Verification items for the finished model (mm, model axes). A direction names the side the tool comes from. Round coordinates to 2 decimals unless told otherwise and drop trailing zeros. One line per item, written item: value. Start each with the question number.
Autodesk Inventor part; units mm, degrees
ref_plane "Work Plane1" through (0, 0, 0.5) normal (0, 0, -1) x (-1, 0, 0)
ref_plane "Work Plane2" through (0, 0, 0.8) normal (0, 0, -1) x (-1, 0, 0)
ref_plane "Work Plane3" through (0, 0, 1.3) normal (0, 0, -1) x (-1, 0, 0)
sketch "Sketch1" plane through (0, 0, 0) normal (0, 0, 1) x (1, 0, 0)
  line L0 (-25, 2) -> (-25, -2)
  line L1 (0, 0.3189) -> (0, -1.0844) construction
  line L2 (-25, 2) -> (25, 2)
  line L3 (25, 2) -> (25, -2)
  line L4 (25, -2) -> (-25, -2)
  line L5 (-1.8046, 0) -> (4.5195, 0) construction
  arc A0 (-23.4, 2) -> (-21.6, 2) centre (-22.5, 2) ccw
  arc A1 (-20.025, 2) -> (-15.975, 2) centre (-18, 2) ccw
  arc A2 (-15.525, 2) -> (-11.475, 2) centre (-13.5, 2) ccw
  arc A3 (-11.025, 2) -> (-6.975, 2) centre (-9, 2) ccw
  arc A4 (-5.4, 2) -> (-3.6, 2) centre (-4.5, 2) ccw
  arc A5 (-2.025, 2) -> (2.025, 2) centre (0, 2) ccw
  arc A6 (2.475, 2) -> (6.525, 2) centre (4.5, 2) ccw
  arc A7 (6.975, 2) -> (11.025, 2) centre (9, 2) ccw
  arc A8 (11.475, 2) -> (15.525, 2) centre (13.5, 2) ccw
  arc A9 (17.125, 2) -> (18.875, 2) centre (18, 2) ccw
  arc A10 (21.625, 2) -> (23.375, 2) centre (22.5, 2) ccw
  arc A11 (-18.225, -2) -> (-22.275, -2) centre (-20.25, -2) ccw
  arc A12 (-13.725, -2) -> (-17.775, -2) centre (-15.75, -2) ccw
  arc A13 (-9.225, -2) -> (-13.275, -2) centre (-11.25, -2) ccw
  arc A14 (-4.725, -2) -> (-8.775, -2) centre (-6.75, -2) ccw
  arc A15 (-2.535, -2) -> (-4.255, -2) centre (-3.395, -2) ccw
  arc A16 (-0.245, -2) -> (-1.965, -2) centre (-1.105, -2) ccw
  arc A17 (4.275, -2) -> (0.225, -2) centre (2.25, -2) ccw
  arc A18 (8.775, -2) -> (4.725, -2) centre (6.75, -2) ccw
  arc A19 (13.275, -2) -> (9.225, -2) centre (11.25, -2) ccw
  arc A20 (17.775, -2) -> (13.725, -2) centre (15.75, -2) ccw
  arc A21 (20.675, -2) -> (18.925, -2) centre (19.8, -2) ccw
  arc A22 (23.375, -2) -> (21.625, -2) centre (22.5, -2) ccw
  point P0 (0, 0)
  dimension "d0" = 4
  dimension "d1" = 50
  dimension "d2" = 2.5
  dimension "d3" = 4.5
  dimension "d4" = 4.5
  dimension "d5" = 4.5
  dimension "d6" = 4.5
  dimension "d7" = 4.5
  dimension "d8" = 4.5
  dimension "d10" = 4.5
  dimension "d11" = 4.5
  dimension "d12" = 4.5
  dimension "d13" = 4.5
  dimension "d14" = 1.8
  dimension "d15" = 4.05
  dimension "d16" = 4.05
  dimension "d17" = 4.05
  dimension "d18" = 1.8
  dimension "d19" = 4.05
  dimension "d20" = 4.05
  dimension "d21" = 4.05
  dimension "d22" = 4.05
  dimension "d23" = 1.75
  dimension "d24" = 1.75
  dimension "d25" = 4.05
  dimension "d27" = 4.5
  dimension "d28" = 4.5
  dimension "d29" = 4.5
  dimension "d30" = 3.355
  dimension "d31" = 2.29
  dimension "d32" = 3.355
  dimension "d33" = 4.5
  dimension "d34" = 4.5
  dimension "d35" = 4.5
  dimension "d37" = 1.75
  dimension "d38" = 4.05
  dimension "d39" = 4.05
  dimension "d40" = 4.05
  dimension "d41" = 4.05
  dimension "d42" = 1.72
  dimension "d43" = 1.72
  dimension "d44" = 4.05
  dimension "d45" = 4.05
  dimension "d46" = 4.05
  dimension "d47" = 1.75
  dimension "d48" = 2.7
  dimension "d136" = 2.5
  dimension "d143" = 4.05
extrude "Extrusion1" add sketch "Sketch1" along normal blind 12 contours L2 A0 A1 A2 A3 A4 A5 A6 A7 A8 A9 A10 L3 L4 A22 A21 A20 A19 A18 A17 A16 A15 A14 A13 A12 A11 L0
sketch "Sketch2" plane through (23.375, 2, 0) normal (0, 1, 0) x (1, 0, 0)
  circle A0 centre (3.025, -9.9997) radius 2
  line L0 (1.625, 0) -> (1.625, -12)
  line L1 (1.625, -12) -> (1.625, -11.428)
  point P0 (-23.375, 0)
  dimension "d51" = 4
  dimension "d52" = 0.572
  dimension "d55" = 1.4
extrude "Extrusion2" cut sketch "Sketch2" against normal blind 12.5
sketch "Sketch3" plane through (-25, 2, 0) normal (0, 1, 0) x (1, 0, 0)
  circle A0 centre (-1.4, -9.9997) radius 2
  line L0 (0, 0) -> (0, -12)
  line L1 (0, -12) -> (0, -11.428)
  point P0 (25, 0)
  dimension "d58" = 4
  dimension "d59" = 0.572
  dimension "d60" = 1.4
extrude "Extrusion3" cut sketch "Sketch3" against normal blind 12.5
sketch "Sketch4" plane through (0, 0, 12) normal (0, 0, 1) x (1, 0, 0)
  line L0 (-22.4782, 2) -> (21.8218, 2)
  line L1 (21.8218, 2) -> (21.8218, 1.825)
  line L2 (21.8218, 1.825) -> (-22.4782, 1.825)
  line L3 (-22.4782, 1.825) -> (-22.4782, 2)
  line L4 (-20.025, 2) -> (-21.6, 2)
  line L5 (-25, 2) -> (-25, -2)
  line L6 (13.275, -2) -> (13.725, -2)
  line L7 (-21.5, -2) -> (-8, -2)
  line L8 (-8, -2) -> (-8, -1.825)
  line L9 (-8, -1.825) -> (-21.5, -1.825)
  line L10 (-21.5, -1.825) -> (-21.5, -2)
  line L11 (0.89, -2) -> (21.8842, -2)
  line L12 (21.8842, -2) -> (21.8842, -1.825)
  line L13 (21.8842, -1.825) -> (0.89, -1.825)
  line L14 (0.89, -1.825) -> (0.89, -2)
  line L15 (-13.725, -2) -> (-13.275, -2)
  line L16 (25, -2) -> (25, 2)
  point P0 (0, 0)
  point P1 (-20.8125, 2)
  point P2 (13.5, -2)
  point P3 (-13.5, -2)
  dimension "d63" = 0.175
  dimension "d64" = 44.3
  dimension "d65" = 2.5218
  dimension "d69" = 0.175
  dimension "d70" = 0.175
  dimension "d71" = 3.5
  dimension "d72" = 17
  dimension "d73" = 3.1158
  dimension "d74" = 24.11
extrude "Extrusion4" cut sketch "Sketch4" against normal blind 12.5
ref_plane "Work Plane1" through (0, 0, 0.5) normal (0, 0, -1) x (-1, 0, 0)
sketch "Sketch5" plane through (0, 0, 0.5) normal (0, 0, -1) x (-1, 0, 0)
  line L0 (25, 2) -> (25, -2)
  line L1 (25, 2) -> (25, 3.5)
  line L2 (25, 3.5) -> (24.5, 3.5)
  line L3 (24.5, 3.5) -> (24.1998, 2.7996)
  line L4 (24.1998, 2.7996) -> (24.3998, 2.7996)
  line L5 (24.3998, 2.7996) -> (24.3998, 2)
  line L6 (23.4, 2) -> (25, 2)
  line L7 (25, -2) -> (22.275, -2)
  line L8 (25, -2) -> (25, -3.5)
  line L9 (25, -3.5) -> (24.5, -3.5)
  line L10 (24.5, -3.5) -> (24.1998, -2.7996)
  line L11 (24.1998, -2.7996) -> (24.3998, -2.7996)
  line L12 (24.3998, -2.7996) -> (24.3998, -2)
  line L13 (0, 0) -> (0, 7.5844) construction
  line L14 (25, 2) -> (24.3998, 2)
  line L15 (25, -2) -> (24.3998, -2)
  line L16 (-25, 2) -> (-25, -2)
  line L17 (-25, 2) -> (-25, 3.5)
  line L18 (-25, 3.5) -> (-24.5, 3.5)
  line L19 (-24.5, 3.5) -> (-24.1998, 2.7996)
  line L20 (-24.1998, 2.7996) -> (-24.3998, 2.7996)
  line L21 (-24.3998, 2.7996) -> (-24.3998, 2)
  line L22 (-23.4, 2) -> (-25, 2)
  line L23 (-25, -2) -> (-22.275, -2)
  line L24 (-25, -2) -> (-25, -3.5)
  line L25 (-25, -3.5) -> (-24.5, -3.5)
  line L26 (-24.5, -3.5) -> (-24.1998, -2.7996)
  line L27 (-24.1998, -2.7996) -> (-24.3998, -2.7996)
  line L28 (-24.3998, -2.7996) -> (-24.3998, -2)
  line L29 (-25, 2) -> (-24.3998, 2)
  line L30 (-25, -2) -> (-24.3998, -2)
  dimension "d78" = 1.5
  dimension "d79" = 0.5
  dimension "d80" = 0.762
  dimension "d81" = 0.2
  dimension "d83" = 113.2
  dimension "d84" = 0.7996
  dimension "d85" = 1.5
  dimension "d86" = 0.5
  dimension "d87" = 113.2
  dimension "d88" = 0.2
  dimension "d89" = 0.762
extrude "Extrusion5" add sketch "Sketch5" against normal blind 6 contours L8 L9 L10 L11 L12 L7 | L6 L5 L4 L3 L2 L1
ref_plane "Work Plane2" through (0, 0, 0.8) normal (0, 0, -1) x (-1, 0, 0)
sketch "Sketch8" plane through (0, 0, 0.8) normal (0, 0, -1) x (-1, 0, 0)
  line L0 (25, 2) -> (25, 3.5)
  line L1 (25, 3.5) -> (24.5, 3.5)
  line L2 (24.5, 3.5) -> (24.1998, 2.7996)
  line L3 (24.1998, 2.7996) -> (24.3998, 2.7996)
  line L4 (24.3998, 2.7996) -> (24.3998, 2)
  line L5 (24.25, 2) -> (25, 2)
  line L6 (25, 2) -> (24.3998, 2)
  arc A0 (-2.0174, 1.825) -> (2.0174, 1.825) centre (0, 2) ccw
  line L7 (0, 2) -> (0, 7.911) construction
  line L8 (-24.25, 2) -> (-25, 2)
  line L9 (-25, 2) -> (-24.3998, 2)
  line L10 (-24.1998, 2.7996) -> (-24.3998, 2.7996)
  line L11 (-24.3998, 2.7996) -> (-24.3998, 2)
  line L12 (-25, 2) -> (-25, 3.5)
  line L13 (-25, 3.5) -> (-24.5, 3.5)
  line L14 (-24.5, 3.5) -> (-24.1998, 2.7996)
  point P0 (0, 0)
  dimension "d112" = 1.5
  dimension "d113" = 0.5
  dimension "d114" = 0.762
  dimension "d115" = 0.2
  dimension "d116" = 113.2
  dimension "d117" = 0.7996
extrude "Extrusion8" add sketch "Sketch8" against normal blind 6 contours L8 L12 L13 L14 L10 L11
mirror "Mirror1" about plane through (0, 0, 0) normal (0, 1, 0) of "Extrusion8"
ref_plane "Work Plane3" through (0, 0, 1.3) normal (0, 0, -1) x (-1, 0, 0)
sketch "Sketch11" plane through (0, 0, 0) normal (0, 0, -1) x (-1, 0, 0)
  line L0 (-25, 2) -> (-24.4, 2)
  line L1 (-23.375, -2) -> (-25, -2)
  line L2 (-25, 2) -> (-24, 2)
  line L3 (-24, 2) -> (-24, -2)
  line L4 (-24, -2) -> (-25, -2)
  line L5 (-25, -2) -> (-25, 2)
  line L6 (25, 2) -> (25, -2)
  line L7 (25, -2) -> (22.275, -2)
  line L8 (25, 2) -> (24, 2)
  line L9 (24, 2) -> (24, -2)
  line L10 (24, -2) -> (25, -2)
  line L11 (25, -2) -> (25, 2)
  point P0 (0, 0)
  dimension "d145" = 1
  dimension "d146" = 1
extrude "Extrusion11" add sketch "Sketch11" along normal blind 2.005
fillet "Fillet1" radius 0.5 2 edges at (24, 0, 0) (-24, 0, 0)
sketch "Sketch12" plane through (0, 0, -2.005) normal (0, 0, -1) x (-1, 0, 0)
  line L0 (-25, 2) -> (-25, -2)
  line L1 (-24, -2) -> (-24, 2)
  line L2 (-25, 0.9) -> (-24, 0.9)
  line L3 (-24, 0.9) -> (-24, -0.8147)
  line L4 (-24, -0.8147) -> (-25, -0.8147)
  line L5 (-25, -0.8147) -> (-25, 0.9)
  line L6 (-24, 2) -> (-25, 2)
  line L7 (-23.375, -2) -> (-25, -2)
  line L8 (-25, -2) -> (-24, -2)
  line L9 (-24, -2) -> (-24, -0.9)
  line L10 (-24, -0.9) -> (-25, -0.9)
  line L11 (-25, -0.9) -> (-25, -2)
  line L12 (25, -2) -> (25, 2)
  line L13 (25, 2) -> (24, 2)
  line L14 (24, 2) -> (24, 0.9)
  line L15 (24, 0.9) -> (25, 0.9)
  line L16 (25, 0.9) -> (25, 2)
  line L17 (25, -2) -> (25, -3.5)
  line L18 (25, -2) -> (24, -2)
  line L19 (24, -2) -> (24, -0.9)
  line L20 (24, -0.9) -> (25, -0.9)
  line L21 (25, -0.9) -> (25, -2)
  point P0 (0, 0)
  dimension "d150" = 1.1
  dimension "d151" = 1.1
  dimension "d152" = 1
  dimension "d153" = 1.1
  dimension "d154" = 1
  dimension "d155" = 1.1
extrude "Extrusion12" add sketch "Sketch12" along normal blind 2 contours L6 L1 L2 L0 | L4 L1 L10 L0 | L10 L1 L7 L0 | L18 L19 L20 L12 | L15 L14 L13 L12
sketch "Sketch13" plane through (25, -2, 8.5714) normal (1, 0, 0) x (0, 0, -1)
  line L0 (12.5764, 0) -> (12.5764, 1.1853)
  line L1 (12.5764, 1.1853) -> (10.5764, 1.1853)
  line L2 (12.5764, 1.2003) -> (12.5764, 1.1853)
  line L3 (119.9448, 1.2) -> (10.5764, 1.2) construction
  line L4 (10.5764, 1.2) -> (12.5764, 1.2)
  line L5 (12.5764, 1.2) -> (12.5764, 1.1)
  line L6 (12.5764, 1.1) -> (10.5764, 1.1)
  line L7 (10.5764, 1.1) -> (10.5764, 1.2)
  point P0 (8.5714, 2)
  dimension "d159" = 0.1
extrude "Extrusion13" cut sketch "Sketch13" against normal blind 10
properties part number "3d_LM - Pinza 3" material "PA12 SLS 3D Print"
1. Depth check by flat-ended pin: pin 1 (0.5 mm diameter, centred on x = -24.5, y = -0.5, fed in from -Z) (3 decimals); pin 2 (1.3 mm diameter, centred on x = 16.5, z = 7, fed in from +Y) (3 decimals); pin 3 (0.9 mm diameter, centred on x = 24.5, y = 3, fed in from -Z). Enter the tip coordinate at first touch or a pass-through.
2. Scan lines: line 1 along X through (y, z) = (1.5, -2); line 2 along X through (y, z) = (2.25, 6); line 3 along Z through (x, y) = (-11, 0.75). Record each from-to range of solid material in increasing order.
3. Draft check along Y on faces 4 (the face through (24.5, -0.9, -3)), 5 (the face through (21, -1.825, 6)), 6 (the face through (24.5, -1.4, -4.005)). Enter one of: released by +Y, released by -Y, zero draft, split by the parting line, or undercut.
4. Tool access check on faces 1 (the face through (-21, 1.825, 6)), 2 (the face through (-24.5, 0.9, -3)), 3 (the face through (-24.7, -2.7, 6.5)). Record the directions out of +Z, -Z, +X, -X, +Y, -Y that give a thin tool (end or side, any length) a straight path to the whole face; none if there is none.
Geometry check:
1. pin 1: stops at z = -2.005
1. pin 2: stops at y = 1.825
1. pin 3: stops at z = 0.8
2. line 1: x = -25 to -24, 24 to 25
2. line 2: x = -25 to -24.4, 24.4 to 25
2. line 3: z = 0 to 12
3. face 4: undercut
3. face 5: released by -Y
3. face 6: zero draft
4. face 1: +Z, -Z, +Y
4. face 2: -Z, +X, -X
4. face 3: +Z, -X, -Y
